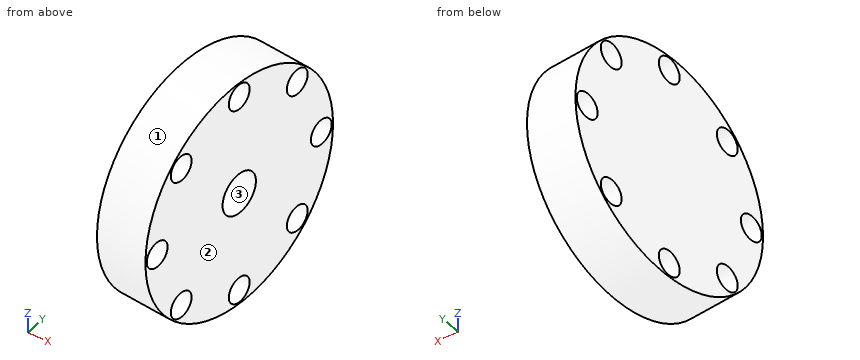
from build123d import *

# Parameters (mm, degrees)
SKETCH1_R           = 14.2875
BOSS_EXTRUDE1_DEPTH = 6.35
SKETCH2_R           = 2.54
CUT_EXTRUDE1_DEPTH  = 5.08
SKETCH3_R           = 1.5875
CUT_EXTRUDE2_DEPTH  = 10


with BuildPart() as part:
    # Sketch1 → Boss-Extrude1 (new body)
    with BuildSketch(Plane(origin=(234.278878836, -18.689027227, 0), x_dir=(0, 0, -1), z_dir=(0.9968332748770866, -0.0795199477981641, 0))):
        with Locations(Location((-43.174261814, 8.550344032, 0), (0, 0, 90))):
            Circle(SKETCH1_R)
    extrude(amount=-BOSS_EXTRUDE1_DEPTH)

    # Sketch2 → Cut-Extrude1 (cut)
    with BuildSketch(Plane(origin=(234.278878836, -18.689027227, 0), x_dir=(0, 0, -1), z_dir=(0.9968332748770866, -0.07951994779816411, 0))):
        with Locations(Location((-43.174261814, 8.550344032, 0), (0, 0, 90))):
            Circle(SKETCH2_R)
    extrude(amount=-CUT_EXTRUDE1_DEPTH, mode=Mode.SUBTRACT)

    # Sketch3 → Cut-Extrude2 (cut)
    with BuildSketch(Plane(origin=(227.94898754, -18.184075559, 0), x_dir=(0, 0, 1), z_dir=(-0.9968332748770866, 0.07951994779816411, 0))):
        with Locations(Location((30.674261814, 8.550344032, 0), (0, 0, 270))):
            Circle(SKETCH3_R)
        with Locations(Location((43.174261814, 21.050344032, 0), (0, 0, 270))):
            Circle(SKETCH3_R)
        with Locations(Location((52.013096579, 17.389178797, 0), (0, 0, 270))):
            Circle(SKETCH3_R)
        with Locations(Location((55.674261814, 8.550344032, 0), (0, 0, 270))):
            Circle(SKETCH3_R)
        with Locations(Location((52.013096579, -0.288490733, 0), (0, 0, 270))):
            Circle(SKETCH3_R)
        with Locations(Location((43.174261814, -3.949655968, 0), (0, 0, 270))):
            Circle(SKETCH3_R)
        with Locations(Location((34.33542705, -0.288490733, 0), (0, 0, 270))):
            Circle(SKETCH3_R)
        with Locations(Location((34.33542705, 17.389178797, 0), (0, 0, 270))):
            Circle(SKETCH3_R)
    extrude(amount=-CUT_EXTRUDE2_DEPTH, mode=Mode.SUBTRACT)


solid = part.part
Input: part model. Units: mm. Frame: model coordinates. Face numbers are marked on the shaded views. Give positions to 0.01 mm unless a question says otherwise; leave off trailing zeros. Order: outer loops, then holes, each group sorted by start corner. A loop starts at its lowest first (then second) coordinate and runs counter-clockwise, first axis right, second up.
Q1. Section B-B on z = 43.75. Output: boundary loops of the cut face in (x, y).
Checked values:
outline: (227.49, -23.89) - (233.82, -24.4) - (233.85, -24.1) - (227.52, -23.6) - close; (227.75, -20.65) - (234.08, -21.15) - (234.76, -12.63) - (229.7, -12.23) - (230.09, -7.3) - (235.16, -7.7) - (235.84, 0.82) - (229.51, 1.32) - close; (229.74, 4.27) - (236.07, 3.77) - (236.09, 4.06) - (229.76, 4.57) - close
Q2. Section C-C on y = -0.25. State how many separate pieces and enclosed holes the cut face has, and give its area (3 significant figures).
Checked values:
separate pieces: 3
enclosed holes: 0
area: 99.9 mm2
Q3. Section A-A on z = 52.5. Output: boundary loops of the cut face in (x, y).
Checked values:
outline: (227.77, -20.45) - (234.1, -20.96) - (234.14, -20.48) - (227.81, -19.98) - close; (228.05, -16.97) - (234.38, -17.47) - (235.54, -2.86) - (229.21, -2.36) - close; (229.45, 0.66) - (235.78, 0.15) - (235.82, 0.62) - (229.49, 1.13) - close
Q4. Ray query, probe 1 along Y at (x, z) = (232.25, 52); probe 2 along Z at (x, y) = (230, -1.5); probe 3 along Z at (x, y) = (232.75, -1). Return the intervals inside material, ascending.
Checked values:
probe 1: y = -21.22 to -20.41, -17.22 to -2.68, 0.51 to 1.32
probe 2: z = 31.51 to 32.86, 35.81 to 50.54, 53.48 to 54.84
probe 3: z = 32.05 to 32.75, 35.92 to 50.43, 53.6 to 54.3
Q5. Draft query along Z for the marked faces 1, 2 and 3. Return one class per face: +Z half, -Z half, draft (parallel to the pull), parting line (faces both ways), or undercut.
Checked values:
face 1: parting line
face 2: draft
face 3: undercut
Q6. Contact query for flat-ended pins moving along their axis: pin 1 Ø1.5 at (y, z) = (-3.5, 38.5) entering from +X; pin 2 Ø2 at (x, z) = (233, 51) entering from +Y; pin 3 Ø1 at (y, z) = (-0.5, 54) entering from -X. Output: stop coordinate, or through.
Checked values:
pin 1: stops at x = 235.55
pin 2: stops at y = 2.59
pin 3: stops at x = 229.32
